CAD build for the part. Positions are in the model's coordinates, mm. Face numbers are marked on the shaded views. Give positions to 0.01 mm unless a question says otherwise; leave off trailing zeros. Write each loop counter-clockwise with the first axis right and the second up, starting at its lowest first coordinate (ties: lowest second). Pieces come first, ordered by that corner, then holes. Notation, with made-up numbers: (51, 74.25) - (95, 74.25) arc R24 ccw to (95, 107.25) - close; hole circle Ø3 at (56.5, -8.5). An arc over 180 degrees is marked (long way). Answer as a JSON object with one key per item and string values.
Autodesk Inventor part; units mm, degrees
ref_plane "YZ Plane" through (0, 0, 0) normal (1, 0, 0) x (0, 1, 0)
ref_plane "XZ Plane" through (0, 0, 0) normal (0, 1, 0) x (-1, 0, 0)
ref_plane "XY Plane" through (0, 0, 0) normal (0, 0, 1) x (1, 0, 0)
sketch "スケッチ1" plane through (0, 0, 0) normal (0, 0, 1) x (1, 0, 0)
  line L0 (44.9825, 3) -> (44.9825, 0)
  line L1 (44.9825, 0) -> (93.5151, 0)
  line L2 (44.9825, 3) -> (93.5151, 3)
  circle A0 centre (152.1179, -73.6808) radius 5
  circle A1 centre (90.7937, -5.925) radius 3
  circle A2 centre (91.5613, -41.579) radius 3
  line L3 (50.9825, 0) -> (47.9825, 0)
  line L4 (47.9825, 0.7) -> (50.9825, 0.7)
  line L5 (-44.9825, -3) -> (-44.9825, 0)
  line L6 (-44.9825, 0) -> (-93.5151, 0)
  line L7 (-44.9825, -3) -> (-93.5151, -3)
  circle A3 centre (-152.1179, 73.6808) radius 5
  circle A4 centre (-90.7937, 5.925) radius 3
  circle A5 centre (-91.5613, 41.579) radius 3
  line L8 (-50.9825, 0) -> (-47.9825, 0)
  line L9 (-47.9825, -0.7) -> (-50.9825, -0.7)
  arc A6 (-39.4825, 0) -> (-39.4825, 78.6808) centre (-39.4825, 39.3404) ccw
  line L10 (-152.1179, 78.6808) -> (-39.4825, 78.6808)
  line L11 (-39.4825, 0) -> (-57.4825, 0)
  line L12 (-147.1179, 78.6808) -> (-147.1179, 73.6808)
  line L13 (-152.1179, 78.6808) -> (-155.1179, 78.6808)
  arc A7 (-39.4825, 0.75) -> (-39.4825, 77.9308) centre (-39.4825, 39.3404) ccw
  line L14 (-39.4825, 0.75) -> (-57.4825, 0.75)
  line L15 (-152.1179, 77.9308) -> (-155.1179, 77.9308)
  line L16 (-39.4825, 77.9308) -> (-152.1179, 77.9308)
  line L17 (-57.4825, 0.75) -> (-57.4825, 0)
  line L18 (-155.1179, 77.9308) -> (-155.1179, 78.6808)
  point P0 (0, 0)
  point P1 (49.4825, 0.7)
  point P2 (-49.4825, -0.7)
  point P3 (0, 0)
  point P4 (-153.6179, 78.6808)
  dimension "d2" = 360
  dimension "d4" = 18
  dimension "d5" = 8
  dimension "d6" = 5
  dimension "d7" = 3
  dimension "d8" = 0.75
  dimension "d42" = 10
extrude "押し出し1" add sketch "スケッチ1" along normal blind 142 contours L6 L17 L14 A7 L16 L12 L10 A6 L11 | L12 L16 A3 L10 | A3 L16 L15 | A3 L15 L18 L13 picked at (-153.5984, 78.0681)
sketch "スケッチ2" plane through (-155.1179, 78.6808, 0) normal (0, 1, 0) x (1, 0, 0)
  line L0 (0, 0) -> (0, -142)
  line L1 (115.6354, 0) -> (0, 0)
  line L2 (115.6354, -142) -> (0, -142)
  line L3 (8, 0) -> (8, -142)
  circle A0 centre (8, -45) radius 1.5
  circle A1 centre (8, -97) radius 1.5
  line L4 (37.6032, 0) -> (72.6032, 0) construction
  line L5 (0, 0) -> (115.6354, 0)
  line L6 (115.6354, 0) -> (115.6354, -15)
  line L7 (115.6354, -15) -> (0, -15)
  line L8 (0, -15) -> (0, 0)
  line L9 (0, -142) -> (115.6354, -142)
  line L10 (115.6354, -142) -> (115.6354, -127)
  line L11 (115.6354, -127) -> (0, -127)
  line L12 (0, -127) -> (0, -142)
  line L13 (115.6354, 0) -> (0, 0)
  line L14 (0, 0) -> (0, -142)
  line L15 (115.6354, -142) -> (0, -142)
  line L16 (115.6354, 0) -> (115.6354, -142)
  line L17 (0, -15) -> (8, -15)
  line L18 (115.6354, 0) -> (115.6354, -142)
  line L19 (0, -30) -> (51.9615, 0)
  line L20 (0, -112) -> (51.9615, -142)
  point P0 (155.1179, 0)
  point P1 (8, -30)
  point P2 (84.9628, 0)
  point P3 (0, -127)
  point P4 (107.627, -142)
  point P5 (0, -19.9913)
  point P6 (25.9808, -127)
  point P7 (25.9808, -15)
  dimension "d12" = 8
  dimension "d13" = 3
  dimension "d14" = 45
  dimension "d15" = 3
  dimension "d16" = 45
  dimension "d28" = 115.6354
  dimension "d29" = 15
  dimension "d30" = 115.6354
  dimension "d31" = 15
  dimension "d32" = 15
  dimension "d33" = 115.6354
  dimension "d34" = 15
  dimension "d35" = 115.6354
  dimension "d36" = 60
  dimension "d37" = 30
  dimension "d38" = 30
  dimension "d39" = 30
extrude "押し出し2" cut sketch "スケッチ2" against normal blind 0.75 contours L1 L3 L7 L0 | L7 L3 L19 L0 | L1 L19 L7 L3 | L7 L19 L3 | L1 L6 L7 L19 | L20 L3 L11 L0 | L11 L3 L2 L0 | L20 L11 L3 | A0 L3 | L3 A0 | L11 L20 L2 L3 | A1 L3 | L3 A1 | L11 L10 L2 L20
sketch "スケッチ4" plane through (-57.4825, 0, 0) normal (0, -1, 0) x (1, 0, 0)
  line L0 (0, 0) -> (18, 0)
  line L1 (18, 0) -> (18, 142)
  line L2 (0, 142) -> (18, 142)
  line L3 (0, 0) -> (0, 142)
  line L4 (8, 142) -> (8, 0)
  circle A0 centre (8, 106.5) radius 1.5
  circle A1 centre (16, 106.5) radius 1.5
  line L5 (0, 71) -> (18, 71)
  line L6 (0, 142) -> (18, 142)
  circle A2 centre (8, 35.5) radius 1.5
  circle A3 centre (16, 35.5) radius 1.5
  line L7 (8, 106.5) -> (16, 106.5)
  point P0 (57.4825, 0)
  dimension "d43" = 8
  dimension "d44" = 3
  dimension "d45" = 35.5
  dimension "d46" = 3
  dimension "d47" = 8
  dimension "d48" = 71
  dimension "d51" = 71
extrude "押し出し4" cut sketch "スケッチ4" against normal blind 0.75 contours A2 L4 | L4 A2 | A1 | A0 L4 | L4 L7 A0 | A0 L7 L4 | A3
equation "\"d32\" = d29"
equation "\"d33\" = d28"
equation "\"d34\" = d31"
equation "\"d35\" = d30"
properties part number "回路BOX背面" material "ポリプロピレン"
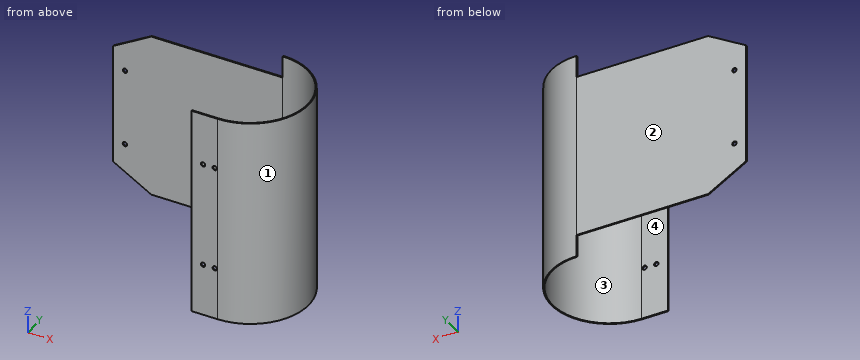
Item 1: Cut at D-D (x = -70). Give the cut face in (y, z).
Entries:
{"outline": "(77.93, 15) - (78.68, 15) - (78.68, 127) - (77.93, 127) - close"}
Item 2: Cut at B-B (z = 133.5). Give the cut face in (x, y), and give its area (3 significant figures).
Entries:
{"outline": "(-57.48, 0) - (-39.48, 0) arc R39.34 ccw to (-39.48, 78.68) - (-39.48, 77.93) arc R38.59 cw to (-39.48, 0.75) - (-57.48, 0.75) - close", "area": "105 mm2"}
Item 3: Cut at A-A (x = -27). Give the cut face in (y, z).
Entries:
{"outline": "(2.03, 0) - (2.82, 0) - (2.82, 142) - (2.03, 142) - close; (75.86, 0) - (76.65, 0) - (76.65, 142) - (75.86, 142) - close"}
Item 4: Flat gauge pins, fed straight in: P1, Ø8, axis at y = 20.5, z = 108.5, coming from the -X side; P2, Ø5, axis at x = -147.12, z = 45, coming from the -Y side; P3, Ø0.8, axis at x = -96.5, y = 78, coming from the -Z side. Where does each tip first touch, or does it go through?
Entries:
{"P1": "x = -8.38", "P2": "y = 77.93", "P3": "z = 15"}
Item 5: Probe line 1 (Y direction, x = -126.5, z = 74.5); line 2 (Y direction, x = -51.5, z = 13); line 3 (Y direction, x = -8.5, z = 79). List the from-to ranges inside material, lowest first. Write a range as from..to.
Entries:
{"line 1": "77.93..78.68", "line 2": "0..0.75", "line 3": "15.1..16.33, 62.35..63.58"}
Item 6: Cut at C-C (y = 67). Give the cut face in (x, z), and give its area (3 significant figures).
Entries:
{"outline": "(-12.57, 0) - (-11.51, 0) - (-11.51, 142) - (-12.57, 142) - close", "area": "151 mm2"}
Item 7: Mould opens along Y. For the marked faces 1, 2, 3 and 4 say: +Y half, -Y half, draft (parallel to the pull), parting line (faces both ways), or undercut.
Entries:
{"face 1": "parting line", "face 2": "+Y half", "face 3": "undercut", "face 4": "undercut"}
